Verification items for the finished model (mm, model axes). A direction names the side the tool comes from. Round coordinates to 2 decimals unless told otherwise and drop trailing zeros. Order: outer loops, then holes, each group sorted by start corner. A loop starts at its lowest first (then second) coordinate and runs counter-clockwise, first axis right, second up. Notation, with made-up numbers: (18.5, 5) -> (59.5, 5) arc R18 cw to (59.5, 25) -> close; hole circle Ø2 at (79, 50.25). An arc over 180 degrees is marked (long way). Return JSON: item names as keys, results as strings. Group by question number.
1) Section check B-B on x = 0. Enter the section's corners in (y, z) (1 decimal), plus the area to 3 significant figures.
2) Depth check by flat-ended pin: pin 1 (1.5 mm diameter, centred on x = -3, y = -10.5, fed in from -Z); pin 2 (1.4 mm diameter, centred on y = 0, z = 7, fed in from -X); pin 3 (1.3 mm diameter, centred on y = -1.5, z = 1.5, fed in from +X). Enter the tip coordinate at first touch or a pass-through.
3) Section check A-A on z = 4.75. Enter the section's corners in (x, y) (1 decimal), plus the area to 3 significant figures.
4) Section check D-D on x = 11.25. Enter the section's corners in (y, z) (1 decimal).
5) Draft check along Y on faces 6 (the cylindrical face through (-3.031, -13.648, 9.37)), 7 (the flat face through (-2.1, -12.4, 8.588)), 8 (the flat face through (0, -2.413, 4)). Enter one of: pulls with the +Y half, pulls with the -Y half, needs draft (parallel to the pull), parting line crosses it, or undercut.
6) Scan lines: L1, parallel to Y at x = -0.25, z = -0.5; L2, parallel to Z at x = 12.5, y = 5 (1 decimal); L3, parallel to Z at x = 7.75, y = -5.5 (3 decimals). Record each from-to range of solid material in increasing order.
7) Tool access check on faces 1 (the flat face through (-1, -1, -1.588)), 2 (the flat face through (3, -3, 0)), 3 (the cylindrical face through (-1.613, 12.287, 5.038)), 4 (the flat face through (0, -3, 10.175)), 5 (the flat face through (-0.845, -2, 4)). Record the directions out of +Z, -Z, +X, -X, +Y, -Y that give a thin tool (end or side, any length) a straight path to the whole face; none if there is none.
```python
from build123d import *

# Parameters (mm, degrees)
F0_R     = 13.97999998
F1_DEPTH = 1.5875
F2_R     = 12.39249998
F3_DEPTH = 7
F4_R     = 13.97999998
F5_DEPTH = 1.5875
F6_R     = 3.96875
F7_DEPTH = 1.5875
F8_W     = 1.56845
F8_H     = 1.6891
F8_W_2   = 1.6891
F8_H_2   = 1.56845
F9_DEPTH = 11.7625


with BuildPart() as f1:
    # F0 (on Top) → F1 (new body)
    with BuildSketch(Plane.XY):
        Circle(F0_R)
    extrude(amount=F1_DEPTH)

    # F2 (on face) → F3 (join)
    with BuildSketch(Plane.XY.offset(1.5875)):
        Circle(F2_R)
    extrude(amount=F3_DEPTH)

    # F4 (on face) → F5 (join)
    with BuildSketch(Plane.XY.offset(8.5875)):
        Circle(F4_R)
    extrude(amount=F5_DEPTH)

    # F6 (on face) → F7 (join)
    with BuildSketch(Plane(origin=(0, 0, 0), x_dir=(1, 0, 0), z_dir=(0, 0, -1))):
        Circle(F6_R)
    extrude(amount=F7_DEPTH)

    # F8 (on face) → F9 (cut, through all)
    with BuildSketch(Plane.XY.offset(10.175)):
        with Locations((1.628775, 0)):
            Rectangle(F8_W, F8_H)
        with Locations((0, -1.628775)):
            Rectangle(F8_W_2, F8_H_2)
        Rectangle(F8_W_2, F8_H)
        with Locations((-1.628775, 0)):
            Rectangle(F8_W, F8_H)
        with Locations((0, 1.628775)):
            Rectangle(F8_W_2, F8_H_2)
    extrude(amount=-F9_DEPTH, mode=Mode.SUBTRACT)


solid = f1.part
```
Check result:
{
 "1": {"outline": "(-14, 0) -> (-4, 0) -> (-4, -1.6) -> (-2.4, -1.6) -> (-2.4, 10.2) -> (-14, 10.2) -> (-14, 8.6) -> (-12.4, 8.6) -> (-12.4, 1.6) -> (-14, 1.6) -> close; (2.4, -1.6) -> (4, -1.6) -> (4, 0) -> (14, 0) -> (14, 1.6) -> (12.4, 1.6) -> (12.4, 8.6) -> (14, 8.6) -> (14, 10.2) -> (2.4, 10.2) -> close", "area": "218 mm^2"},
 "2": {"pin 1": "z = 0", "pin 2": "x = -12.39", "pin 3": "x = 13.95"},
 "3": {"outline": "circle Ø24.8 at (0, 0); hole (-2.4, -0.8) -> (-0.8, -0.8) -> (-0.8, -2.4) -> (0.8, -2.4) -> (0.8, -0.8) -> (2.4, -0.8) -> (2.4, 0.8) -> (0.8, 0.8) -> (0.8, 2.4) -> (-0.8, 2.4) -> (-0.8, 0.8) -> (-2.4, 0.8) -> close", "area": "469 mm^2"},
 "4": {"outline": "(-8.3, 0) -> (8.3, 0) -> (8.3, 1.6) -> (5.2, 1.6) -> (5.2, 8.6) -> (8.3, 8.6) -> (8.3, 10.2) -> (-8.3, 10.2) -> (-8.3, 8.6) -> (-5.2, 8.6) -> (-5.2, 1.6) -> (-8.3, 1.6) -> close"},
 "5": {"face 6": "parting line crosses it", "face 7": "needs draft", "face 8": "undercut"},
 "6": {"L1": "-3.96 to -2.41, 2.41 to 3.96", "L2": "0 to 1.6, 8.6 to 10.2", "L3": "0 to 10.175"},
 "7": {"face 1": "-Z, +X, -X, +Y, -Y", "face 2": "-Z", "face 3": "none", "face 4": "+Z, +X, -X, +Y, -Y", "face 5": "+Z, -Z"}
}
